Input: part model. Units: mm. Frame: model coordinates. Face numbers are marked on the shaded views. A direction names the side the tool comes from. Coordinates: 2 decimals unless noted, no trailing zeros. Order: outer loops, then holes, each group sorted by start corner. A loop starts at its lowest first (then second) coordinate and runs counter-clockwise, first axis right, second up. Notation, with made-up numbers: M -13,73.25 L 4,73.25 A27 cw 4,96.25 Z; hole C 28,17 d3. An arc over 180 degrees is marked long. Answer in a Markdown table with one row per item.
from build123d import *

# Parameters (mm, degrees)
SKETCH2_W           = 41
SKETCH2_H           = 56
SKETCH2_W_2         = 35
SKETCH2_H_2         = 50
BOSS_EXTRUDE1_DEPTH = 20
SKETCH2_3_R         = 65
SKETCH2_3_W         = 41
SKETCH2_3_H         = 56
BOSS_EXTRUDE2_DEPTH = 10
BOSS_EXTRUDE3_DEPTH = 10
SKETCH10_W          = 50
SKETCH10_H          = 2.212003264
CUT_EXTRUDE1_DEPTH  = 10
CUT_EXTRUDE2_START  = 65
SKETCH12_R          = 1.825
CUT_EXTRUDE2_DEPTH  = 11
CIRPATTERN1_COUNT   = 8


with BuildPart() as part:
    # Sketch2 → Boss-Extrude1 (new body)
    with BuildSketch(Plane(origin=(0, 0, 0), x_dir=(1, 0, 0), z_dir=(0, 1, 0))):
        Rectangle(SKETCH2_W, SKETCH2_H)
        Rectangle(SKETCH2_W_2, SKETCH2_H_2, mode=Mode.SUBTRACT)
    extrude(amount=BOSS_EXTRUDE1_DEPTH)

    # Sketch2_3 → Boss-Extrude2 (add)
    with BuildSketch(Plane(origin=(0, 0, 0), x_dir=(1, 0, 0), z_dir=(0, 1, 0))):
        with Locations(Location((0, 0, 0), (0, 0, 270))):
            Circle(SKETCH2_3_R)
        Rectangle(SKETCH2_3_W, SKETCH2_3_H, mode=Mode.SUBTRACT)
    extrude(amount=BOSS_EXTRUDE2_DEPTH)

    # Sketch2_4 → Boss-Extrude3 (add)
    with BuildSketch(Plane(origin=(0, 0, 0), x_dir=(1, 0, 0), z_dir=(0, 1, 0))):
        with BuildLine():
            Line((-17.5, 25), (-17.5, 0))
            Line((-17.5, 0), (-11, 0))
            ThreePointArc((-11, 0), (-7.778174593, 7.778174593), (0, 11))
            Line((0, 11), (0, 25))
            Line((0, 25), (-17.5, 25))
        make_face()
        with BuildLine():
            Line((11, 0), (17.5, 0))
            Line((17.5, 0), (17.5, 25))
            Line((17.5, 25), (0, 25))
            Line((0, 25), (0, 11))
            ThreePointArc((0, 11), (7.778174593, 7.778174593), (11, 0))
        make_face()
        with BuildLine():
            Line((-17.5, 0), (-17.5, -25))
            Line((-17.5, -25), (17.5, -25))
            Line((17.5, -25), (17.5, 0))
            Line((17.5, 0), (11, 0))
            ThreePointArc((11, 0), (0, -11), (-11, 0))
            Line((-11, 0), (-17.5, 0))
        make_face()
    extrude(amount=BOSS_EXTRUDE3_DEPTH)

    # Sketch10 → Cut-Extrude1 (cut)
    with BuildSketch(Plane.ZY.offset(20.5)):
        with Locations((0, 18.893998368)):
            Rectangle(SKETCH10_W, SKETCH10_H)
    extrude(amount=-CUT_EXTRUDE1_DEPTH, mode=Mode.SUBTRACT)

    # Sketch12 → Cut-Extrude2 (cut)
    with BuildSketch(Plane.XY.offset(CUT_EXTRUDE2_START)):
        with Locations((0, 5)):
            Circle(SKETCH12_R)
    cut_extrude2 = extrude(amount=-CUT_EXTRUDE2_DEPTH, mode=Mode.SUBTRACT)

    # CirPattern1: Cut-Extrude2 ×8 about axis
    cirpattern1_axis = Axis((0, 0, 0), (0, 1, 0))
    for i in range(1, CIRPATTERN1_COUNT):
        add(cut_extrude2.rotate(cirpattern1_axis, i * 360 / CIRPATTERN1_COUNT), mode=Mode.SUBTRACT)


solid = part.part
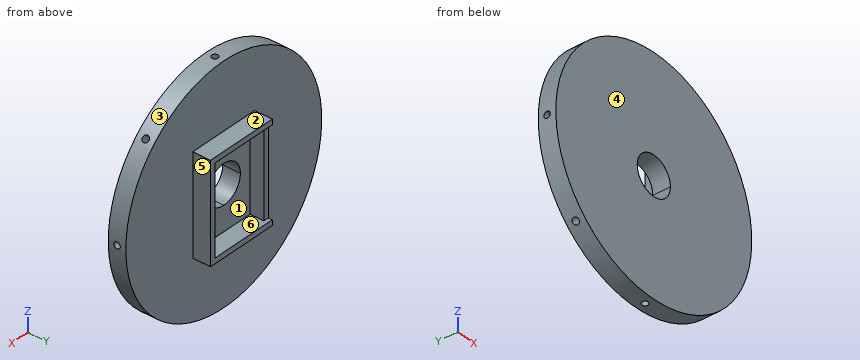
1) Cut plane D-D, the plane z = 52.5. Output: boundary loops of the cut face in (x, y).
Resolved:
| item | result |
|---|---|
| outline | M -38.32,0 L 38.32,0 L 38.32,10 L -38.32,10 Z |
2) Material intervals for probe 1 along Y at (x, z) = (44.5, -44); probe 2 along Y at (x, z) = (34.5, 48); probe 3 along X at (y, z) = (16.5, -23), sorted ascending.
Resolved:
| item | result |
|---|---|
| probe 1 | y = 0 to 3.21, 6.79 to 10 |
| probe 2 | y = 0 to 10 |
| probe 3 | x = -20.5 to -17.5, 17.5 to 20.5 |
3) Cut plane A-A, the plane y = 12.5. Output: boundary loops of the cut face in (x, z), and give its area (3 significant figures).
Resolved:
| item | result |
|---|---|
| outline | M -20.5,-28 L 20.5,-28 L 20.5,28 L -20.5,28 Z; hole M -17.5,-25 L 17.5,-25 L 17.5,25 L -17.5,25 Z |
| area | 546 mm2 |
4) Cut plane B-B, the plane z = -8. Output: boundary loops of the cut face in (x, y).
Resolved:
| item | result |
|---|---|
| outline | M -64.51,0 L -7.55,0 L -7.55,10 L -17.5,10 L -17.5,17.79 L -20.5,17.79 L -20.5,10 L -64.51,10 Z; M 7.55,0 L 64.51,0 L 64.51,10 L 20.5,10 L 20.5,20 L 17.5,20 L 17.5,10 L 7.55,10 Z |
5) Mould query, pull axis X, two halves, no side actions, for the marked faces 4, 5 and 6. Classes: +X half, -X half, draft (parallel to the pull), parting line (faces both ways), or undercut.
Resolved:
| item | result |
|---|---|
| face 4 | draft |
| face 5 | +X half |
| face 6 | undercut |
6) Cut plane C-C, the plane x = -29.5. Output: boundary loops of the cut face in (y, z), and give its area (3 significant figures).
Resolved:
| item | result |
|---|---|
| outline | M 0,-57.92 L 10,-57.92 L 10,57.92 L 0,57.92 Z |
| area | 1,160 mm2 |
7) Reachability of the marked faces 1, 2 and 3 from +Z, -Z, +X, -X, +Y, -Y: full face, straight path, thin tool, end or side. Return the list, or none.
Resolved:
| item | result |
|---|---|
| face 1 | +Y |
| face 2 | +Z, +X, -X, +Y |
| face 3 | +Y, -Y |
8) Contact query for flat-ended pins moving along their axis: pin 1 (2.5 mm diameter, centred on y = 12.5, z = 4.5, fed in from +X); pin 2 (10.5 mm diameter, centred on x = -3, z = -10.5, fed in from +Y); pin 3 (8 mm diameter, centred on y = 13, z = -2, fed in from +X); pin 4 (4 mm diameter, centred on x = 0.5, y = 5, fed in from +Z). Output: stop coordinate, or through.
Resolved:
| item | result |
|---|---|
| pin 1 | stops at x = 20.5 |
| pin 2 | stops at y = 10 |
| pin 3 | stops at x = 65 |
| pin 4 | stops at z = 65 |
